Part model, mm, in its own coordinate system. A direction names the side the tool comes from. Give positions to 0.01 mm unless a question says otherwise; leave off trailing zeros. Order: outer loops, then holes, each group sorted by start corner. A loop starts at its lowest first (then second) coordinate and runs counter-clockwise, first axis right, second up. Notation, with made-up numbers: (76, 65.25) - (112, 65.25) arc R14 cw to (112, 90.25) - close; hole circle Ø11 at (-27.75, 31). An arc over 180 degrees is marked (long way). One line per item, written item: value.
```python
from build123d import *

# Parameters (mm, degrees)
SKETCH1_R           = 3.45
BOSS_EXTRUDE1_DEPTH = 4.2
BOSS_EXTRUDE2_DEPTH = 1.3
SKETCH2_R           = 2.05
CUT_EXTRUDE1_DEPTH  = 0.5
SKETCH4_R           = 0.5
CUT_EXTRUDE2_DEPTH  = 5.2
SKETCH5_R           = 1
CUT_EXTRUDE3_DEPTH  = 4.7
SKETCH6_R           = 2.5
CUT_EXTRUDE4_DEPTH  = 2.6


with BuildPart() as part:
    # Sketch1 → Boss-Extrude1 (new body)
    with BuildSketch(Plane(origin=(0, 0, 0), x_dir=(1, 0, 0), z_dir=(0, 1, 0))):
        Circle(SKETCH1_R)
    extrude(amount=BOSS_EXTRUDE1_DEPTH)

    # Sketch3 → Boss-Extrude2 (add)
    with BuildSketch(Plane(origin=(0, 4.2, 0), x_dir=(1, 0, 0), z_dir=(0, 1, 0))):
        with BuildLine():
            Line((-3.426709786, -0.4002), (-1.986498427, -12.732))
            ThreePointArc((-1.986498427, -12.732), (0, -14.5), (1.986498427, -12.732))
            Line((1.986498427, -12.732), (3.426709786, -0.4002))
            ThreePointArc((3.426709786, -0.4002), (0, 3.45), (-3.426709786, -0.4002))
        make_face()
    extrude(amount=-BOSS_EXTRUDE2_DEPTH)

    # Sketch2 → Cut-Extrude1 (cut)
    with BuildSketch(Plane(origin=(0, 4.2, 0), x_dir=(1, 0, 0), z_dir=(0, 1, 0))):
        Circle(SKETCH2_R)
    extrude(amount=-CUT_EXTRUDE1_DEPTH, mode=Mode.SUBTRACT)

    # Sketch4 → Cut-Extrude2 (cut, through all)
    with BuildSketch(Plane(origin=(0, 4.2, 0), x_dir=(1, 0, 0), z_dir=(0, 1, 0))):
        with Locations((0, -12.5)):
            Circle(SKETCH4_R)
        with Locations((0, -10.625)):
            Circle(SKETCH4_R)
        with Locations((0, -8.75)):
            Circle(SKETCH4_R)
        with Locations((0, -6.875)):
            Circle(SKETCH4_R)
        with Locations((0, -5)):
            Circle(SKETCH4_R)
    extrude(amount=-CUT_EXTRUDE2_DEPTH, mode=Mode.SUBTRACT)

    # Sketch5 → Cut-Extrude3 (cut, through all)
    with BuildSketch(Plane(origin=(0, 3.7, 0), x_dir=(1, 0, 0), z_dir=(0, 1, 0))):
        Circle(SKETCH5_R)
    extrude(amount=-CUT_EXTRUDE3_DEPTH, mode=Mode.SUBTRACT)

    # Sketch6 → Cut-Extrude4 (cut)
    with BuildSketch(Plane.XZ):
        Circle(SKETCH6_R)
    extrude(amount=-CUT_EXTRUDE4_DEPTH, mode=Mode.SUBTRACT)


solid = part.part
```
1) Cut at A-A, the plane z = 5. Give the cut face in (x, y), then the cut area to 3 significant figures.
Outcome:
outline: (-2.89, 2.9) - (-0.5, 2.9) - (-0.5, 4.2) - (-2.89, 4.2) - close; (0.5, 2.9) - (2.89, 2.9) - (2.89, 4.2) - (0.5, 4.2) - close
area: 6.21 mm^2
2) Mould opens along Z. For faces 1 (the cylindrical face through (0, 3.6, 14.5)), 2 (the cylindrical face through (-0.065, 3.559, 4.504)), 3 (the flat face through (1, 2.9, 7)) say: released by +Z, released by -Z, zero draft, split by the parting line, or undercut.
Outcome:
face 1: released by +Z
face 2: undercut
face 3: zero draft
3) Pin check, flat tips, straight feed: pin 1 (1.6 mm diameter, centred on x = 0, z = 0, fed in from -Y); pin 2 (3.5 mm diameter, centred on x = 0, z = 0, fed in from +Y); pin 3 (3.5 mm diameter, centred on x = 0.5, z = 10, fed in from -Y); pin 4 (1.5 mm diameter, centred on x = -2, y = 2, fed in from -Z). Stop position of each tip, or through.
Outcome:
pin 1: passes through
pin 2: stops at y = 3.7
pin 3: stops at y = 2.9
pin 4: stops at z = -3.22
4) Drill centre lines: line 1 along Y through (x, z) = (-0.75, 4.5); line 2 along Z through (x, y) = (0, 1.35); line 3 along Z through (x, y) = (-1.5, 1.2). Where is each one in solid material? Low to high. Write a range as from..to.
Outcome:
line 1: y = 2.9..4.2
line 2: z = -3.45..-2.5, 2.5..3.45
line 3: z = -3.11..-2, 2..3.11
5) Which spindle directions (+Z, -Z, +X, -X, +Y, -Y) get a long thin tool onto all of the face, cutting with end or side? Do faces 4 (the cylindrical face through (-0.267, 3.954, -2.033)), 5 (the cylindrical face through (0, 4, 13)), 6 (the cylindrical face through (-0.54, 1.28, -2.44)). Say none if no direction does.
Outcome:
face 4: +Y
face 5: +Y, -Y
face 6: -Y
6) Cut at B-B, the plane y = 0.8. Give the cut face in (x, z), then the cut area to 3 significant figures.
Outcome:
outline: circle Ø6.9 at (0, 0); hole circle Ø5 at (0, 0)
area: 17.8 mm^2
7) Cut at C-C, the plane x = 0. Give the number of separate pieces and of enclosed holes in the cut face, then the cut area to 3 significant figures.
Outcome:
separate pieces: 7
enclosed holes: 0
area: 19.6 mm^2
8) Cut at D-D, the plane z = 3. Give the cut face in (x, y), then the cut area to 3 significant figures.
Outcome:
outline: (-3.12, 2.9) - (-1.7, 2.9) - (-1.7, 0) - (1.7, 0) - (1.7, 2.9) - (3.12, 2.9) - (3.12, 4.2) - (-3.12, 4.2) - close
area: 18.0 mm^2
